Could you check a few things on this model? Use its own coordinates, in mm. Face numbers are marked on the shaded views. Give positions to 0.01 mm unless a question says otherwise; leave off trailing zeros. Order: outer loops, then holes, each group sorted by start corner. A loop starts at its lowest first (then second) coordinate and runs counter-clockwise, first axis right, second up. Notation, with made-up numbers: M 86.5,29.5 L 140.5,29.5 A7 ccw 140.5,37.5 Z; hole C -2.75,-14 d1. An arc over 180 degrees is marked long. Return JSON: item names as keys, results as strings. Group by question number.
```python
from build123d import *

# Parameters (mm, degrees)
F0_W     = 165.1
F0_H     = 203.2
F0_R     = 1.27
F1_DEPTH = 7.62
F2_W     = 165.1
F2_H     = 38.1
F2_W_2   = 48.26
F2_H_2   = 20.32
F3_DEPTH = 5.08
F6_DEPTH = 5.08
F7_W     = 88.9
F7_H     = 25.4
F7_R     = 6.35
F8_DEPTH = 5.08


with BuildPart() as f1:
    # F0 (on Top) → F1 (new body)
    with BuildSketch(Plane.XY):
        Rectangle(F0_W, F0_H)
        with Locations((-39.6875, -76.835)):
            Circle(F0_R, mode=Mode.SUBTRACT)
        with Locations((-20.6375, -85.725)):
            Circle(F0_R, mode=Mode.SUBTRACT)
        with Locations((-19.3675, -37.465)):
            Circle(F0_R, mode=Mode.SUBTRACT)
        with Locations((31.4325, -80.645)):
            Circle(F0_R, mode=Mode.SUBTRACT)
        with Locations((39.6875, -76.835)):
            Circle(F0_R, mode=Mode.SUBTRACT)
        with Locations((31.4325, -52.705)):
            Circle(F0_R, mode=Mode.SUBTRACT)
        with Locations((-39.6875, 10.16)):
            Circle(F0_R, mode=Mode.SUBTRACT)
        with Locations((39.6875, 10.16)):
            Circle(F0_R, mode=Mode.SUBTRACT)
    extrude(amount=F1_DEPTH)

    # F4: F3 across plane


with BuildPart() as f3:
    # F2 (on face) → F3 (new body)
    with BuildSketch(Plane.YZ.offset(82.55)):
        with Locations((-19.05, -19.05)):
            Rectangle(F2_W, F2_H)
        with Locations((-58.42, -19.685)):
            Rectangle(F2_W_2, F2_H_2, mode=Mode.SUBTRACT)
        Polygon((101.6, 0), (63.5, 0), (63.5, -38.1), align=None)
    extrude(amount=-F3_DEPTH)


with BuildPart() as f1_1:
    add(f1.part)
    add(f3.part.mirror(Plane.YZ))


    add(f3.part)  # F6 merges F3
    # F5 (on face) → F6 (join)
    with BuildSketch(Plane(origin=(0, 101.6, 0), x_dir=(-1, 0, 0), z_dir=(0, 1, 0))):
        Polygon((77.47, 0), (-82.55, 0), (-44.45, -38.1), (44.45, -38.1), (82.55, 0), align=None)
    extrude(amount=-F6_DEPTH)

    # F7 (on face) → F8 (join)
    with BuildSketch(Plane(origin=(0, 0, -38.1), x_dir=(1, 0, 0), z_dir=(0, 0, -1))):
        with Locations((0, -83.82)):
            Rectangle(F7_W, F7_H)
        with Locations((0, -83.82)):
            Circle(F7_R, mode=Mode.SUBTRACT)
    extrude(amount=-F8_DEPTH)


solid = f1_1.part
```
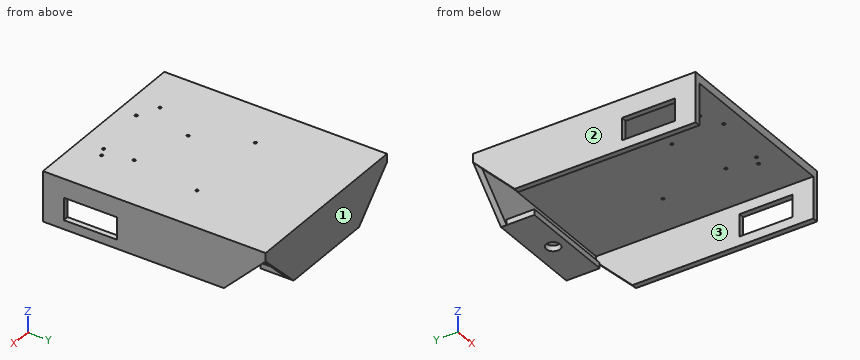
1. Imagine slicing it at C-C, the plane x = 0. Please give me the cut outline in (y, z).
2. I need wall thicknesses on L1, parallel to X at y = -56.5, z = -4; L2, parallel to X at y = 83.82, z = -36.4; L3, parallel to Y at x = 41, z = -14. Which ranges of each line are inside material? Lowest first, please. Write a range as from..to.
3. Imagine slicing it at A-A, the plane y = -67. Please give me the cut outline in (x, z) (3 decimals).
4. Imagine slicing it at B-B, the plane z = -27.5. Please give me the cut outline in (x, y), plus the area to 3 significant figures.
5. Imagine slicing it at D-D, the plane z = -2.5. Please give me the cut outline in (x, y), plus the area to 3 significant figures.
6. For pin 1 (5.5 mm diameter, centred on x = 79.5, z = -21.5, fed in from +Y); pin 2 (6 mm diameter, centred on x = -17, z = -9, fed in from -Y); pin 3 (1.5 mm diameter, centred on y = 78, z = -34.5, fed in from +X), each with a flat end and sliding along its axis, tell me the tip position at first contact or that it passes through.
7. If we mould it in two halves opening along X, with no side actions, what happens to the marked faces 1, 2 and 3? For each: pulls with the +X half, pulls with the -X half, needs draft (parallel to the pull), parting line crosses it, or undercut.
Values:
{
 "1": {"outline": "M -101.6,0 L 96.52,0 L 96.52,-33.02 L 90.17,-33.02 L 90.17,-38.1 L 101.6,-38.1 L 101.6,7.62 L -101.6,7.62 Z; M 71.12,-38.1 L 77.47,-38.1 L 77.47,-33.02 L 71.12,-33.02 Z"},
 "2": {"L1": "x = -82.55..-77.47, 77.47..82.55", "L2": "x = -44.45..-6.35, 6.35..44.45", "L3": "y = 96.52..101.6"},
 "3": {"outline": "M -82.55,-38.1 L -77.47,-38.1 L -77.47,-29.845 L -82.55,-29.845 Z; M -82.55,-9.525 L -77.47,-9.525 L -77.47,0 L 77.47,0 L 77.47,-9.525 L 82.55,-9.525 L 82.55,7.62 L -82.55,7.62 Z; M 77.47,-38.1 L 82.55,-38.1 L 82.55,-29.845 L 77.47,-29.845 Z"},
 "4": {"outline": "M -82.55,-101.6 L -77.47,-101.6 L -77.47,-82.55 L -82.55,-82.55 Z; M -82.55,-34.29 L -77.47,-34.29 L -77.47,74.1 L -82.55,74.1 Z; M -55.05,96.52 L 55.05,96.52 L 55.05,101.6 L -55.05,101.6 Z; M 77.47,-101.6 L 82.55,-101.6 L 82.55,-82.55 L 77.47,-82.55 Z; M 77.47,-34.29 L 82.55,-34.29 L 82.55,74.1 L 77.47,74.1 Z", "area": "1,850 mm²"},
 "5": {"outline": "M -82.55,-101.6 L -77.47,-101.6 L -77.47,96.52 L 77.47,96.52 L 77.47,-101.6 L 82.55,-101.6 L 82.55,99.1 L 80.05,99.1 L 80.05,101.6 L -80.05,101.6 L -80.05,99.1 L -82.55,99.1 Z", "area": "2,840 mm²"},
 "6": {"pin 1": "stops at y = 82.85", "pin 2": "stops at y = 96.52", "pin 3": "stops at x = 44.45"},
 "7": {"face 1": "needs draft", "face 2": "pulls with the -X half", "face 3": "undercut"}
}
